Solid Edge part; units mm, degrees
sketch "Sketch1" plane through (0, 0, 0) normal (0, 0, 1) x (1, 0, 0)
  circle A0 centre (0, 0) radius 40
extrude "Protrusion1" add sketch "Sketch1" along normal blind 12
hole "Bohrung_1" at (0, 0, 12) direction (0, 0, -1) diameter 20 end through all
sketch "Sketch2" plane through (0, 0, 0) normal (0, 0, 1) x (1, 0, 0)
  line L0 (-37.081, 15) -> (-37.081, -15)
extrude "Cutout1" cut sketch "Sketch2" along normal through all material side at (-37.131, 0, 0)
sketch "Sketch3" plane through (-37.081, 0, 6) normal (-1, 0, 0) x (0, -1, 0)
  line L0 (14.4, 4) -> (-14.4, 4)
  line L1 (-14.4, 4) -> (-14.4, -4)
  line L2 (-14.4, -4) -> (14.4, -4)
  line L3 (14.4, -4) -> (14.4, 4)
extrude "Extrusionsausschnitt_5" cut sketch "Sketch3" against normal blind 25
sketch "Sketch4" plane through (-24.581, 0, 2) normal (0, 0, 1) x (0, -1, 0)
  line L0 (-7.75, 7.5) -> (-7.75, -7.5)
  line L1 (-7.75, -7.5) -> (-10.75, -7.5)
  line L2 (-10.75, -7.5) -> (-10.75, 7.5)
  line L3 (-10.75, 7.5) -> (-7.75, 7.5)
extrude "Cutout2" cut sketch "Sketch4" against normal through all
mirror "Mirror1" about plane through (0, 0, 0) normal (0, -1, 0) of "Cutout2"
pattern_circular "Pattern1" count 3 over 360 about axis through (0, 0, 0) along (0, 0, -1) of "Mirror1", "Cutout2", "Extrusionsausschnitt_5", "Cutout1"
Read the model definition and answer for the solid it produces. Units are mm, in the model's axes. A direction names the side the tool comes from. Round coordinates to 2 decimals unless told otherwise and drop trailing zeros. Write each loop counter-clockwise with the first axis right and the second up, starting at its lowest first coordinate (ties: lowest second). Pieces come first, ordered by that corner, then holes. Notation, with made-up numbers: (-30.75, -27.75) - (-26.75, -27.75) arc R19 ccw to (-26.75, 5.25) - close; hole circle Ø9 at (23, -7). An arc over 180 degrees is marked (long way). Use a Markdown table: item, result.
(1) The part is cut by section B-B (z = 7.75). Write down the section's boundary in (x, y).
Reported:
| item | result |
|---|---|
| outline | (-37.08, -15) arc R40 ccw to (5.55, -39.61) - (6.07, -39.31) - (-6.43, -17.66) - (18.51, -3.26) - (31.01, -24.91) - (31.53, -24.61) arc R40 ccw to (31.53, 24.61) - (31.01, 24.91) - (18.51, 3.26) - (-6.43, 17.66) - (6.07, 39.31) - (5.55, 39.61) arc R40 ccw to (-37.08, 15) - (-37.08, 14.4) - (-12.08, 14.4) - (-12.08, -14.4) - (-37.08, -14.4) - close; hole circle Ø20 at (0, 0) |
(2) Straight lines are drawn through the part: line 1 along Z through (x, y) = (-22, 2); line 2 along Y through (x, z) = (2.5, 1); line 3 along X through (y, z) = (0, 9.25). For each, find the intervals that lie inside material, in ascending order. Write a range as [from, to].
Reported:
| item | result |
|---|---|
| line 1 | [0, 2], [10, 12] |
| line 2 | [-39.92, -25.83], [-19.83, -9.68], [9.68, 19.83], [25.83, 39.92] |
| line 3 | [-12.08, -10], [10, 40] |
(3) The part is cut by section C-C (y = 26.5). Write down the section's boundary in (x, z).
Reported:
| item | result |
|---|---|
| outline | (-29.96, 0) - (2.89, 0) - (2.89, 2) - (-1.33, 2) - (-1.33, 10) - (28.26, 10) - (28.26, 12) - (-29.96, 12) - close; (6.35, 0) - (28.26, 0) - (28.26, 2) - (6.35, 2) - close |
(4) Each of these flat-tipped pins is pushed along its axis until it touches: pin 1 Ø11 at (x, y) = (13, 19.5) entering from -Z; pin 2 Ø0.6 at (y, z) = (9, 1) entering from +X; pin 3 Ø3 at (y, z) = (-0.5, 4.5) entering from -X; pin 4 Ø2 at (x, z) = (1.5, 1) entering from +Y. Where does it stop, or does it pass through?
Reported:
| item | result |
|---|---|
| pin 1 | z = 0 |
| pin 2 | x = 39.04 |
| pin 3 | x = -12.08 |
| pin 4 | y = 40 |
(5) Which of the six approach directions +Z, -Z, +X, -X, +Y, -Y give full straight-line access (tool end or side, diameter ignored) to faces 5 (the flat face through (9, -8, 0)), 6 (the flat face through (-25, -7.75, 1)), 7 (the flat face through (12, -22, 2)), 8 (the flat face through (-12.081, 0, 6))?
Reported:
| item | result |
|---|---|
| face 5 | -Z, +X, -X, +Y, -Y |
| face 6 | -Z |
| face 7 | none |
| face 8 | -X |
(6) The part is cut by section A-A (y = 0). Write down the section's boundary in (x, z).
Reported:
| item | result |
|---|---|
| outline | (-37.08, 0) - (-10, 0) - (-10, 12) - (-37.08, 12) - (-37.08, 10) - (-12.08, 10) - (-12.08, 2) - (-37.08, 2) - close; (10, 0) - (40, 0) - (40, 12) - (10, 12) - close |
(7) The mould has two halves that part along Z. Classify faces 1 (the flat face through (13, 21, 2)), 2 (the flat face through (-25, -14.4, 6)), 3 (the flat face through (-8, -8, 12)), 4 (the flat face through (-17.081, -9, 1)): released by +Z, released by -Z, zero draft, split by the parting line, or undercut.
Reported:
| item | result |
|---|---|
| face 1 | undercut |
| face 2 | undercut |
| face 3 | released by +Z |
| face 4 | zero draft |
